```python
from build123d import *

# Parameters (mm, degrees)
SKETCH1_W                           = 250
SKETCH1_H                           = 250
SKETCH1_W_2                         = 4.8
SKETCH1_H_2                         = 20
SKETCH1_W_3                         = 10
SKETCH1_H_3                         = 2.9
SKETCH1_W_4                         = 2.9
SKETCH1_H_4                         = 30
SKETCH1_H_5                         = 50
SKETCH1_W_5                         = 6
SKETCH1_H_6                         = 70
BOSS_EXTRUDE1_DEPTH                 = 2
SKETCH2_R                           = 2.5
CUT_EXTRUDE1_DEPTH                  = 3
SKETCH3_R                           = 3.25
CUT_EXTRUDE2_DEPTH                  = 3
SKETCH4_W                           = 2
SKETCH4_H                           = 20
SKETCH4_W_2                         = 20
SKETCH4_H_2                         = 2
BOSS_EXTRUDE2_DEPTH                 = 2
F_4_5_4_5_DIAMETER_HOLE1_AT_2_COUNT = 2
F_4_5_4_5_DIAMETER_HOLE1_AT_2_PITCH = 50
F_4_5_4_5_DIAMETER_HOLE1_AT_3_COUNT = 2
F_4_5_4_5_DIAMETER_HOLE1_AT_3_PITCH = 130
F_4_5_4_5_DIAMETER_HOLE1_AT_4_COUNT = 2
F_4_5_4_5_DIAMETER_HOLE1_AT_4_PITCH = 120
SKETCH9_W                           = 4.8
SKETCH9_H                           = 20
CUT_EXTRUDE3_DEPTH                  = 3
SKETCH10_R                          = 2.1
CUT_EXTRUDE4_DEPTH                  = 5
SKETCH_1_R                          = 2.25
CUT_EXTRUDE_1_DEPTH                 = 2
CUT_EXTRUDE_1_DEPTH_BACK            = 10


with BuildPart() as part:
    # Sketch1 → Boss-Extrude1 (new body)
    with BuildSketch(Plane(origin=(0, 0, 0), x_dir=(1, 0, 0), z_dir=(0, 1, 0))):
        with Locations((125, 125)):
            Rectangle(SKETCH1_W, SKETCH1_H)
        with Locations((142.5, 15)):
            Rectangle(SKETCH1_W_2, SKETCH1_H_2, mode=Mode.SUBTRACT)
        with Locations((107.5, 15)):
            Rectangle(SKETCH1_W_2, SKETCH1_H_2, mode=Mode.SUBTRACT)
        with Locations((92, 53.93422616)):
            Rectangle(SKETCH1_W_3, SKETCH1_H_3, mode=Mode.SUBTRACT)
        with Locations((103.55, 79.434226159)):
            Rectangle(SKETCH1_W_4, SKETCH1_H_4, mode=Mode.SUBTRACT)
        with Locations((92, 104.93422616)):
            Rectangle(SKETCH1_W_3, SKETCH1_H_3, mode=Mode.SUBTRACT)
        with Locations((107.5, 125)):
            Rectangle(SKETCH1_W_2, SKETCH1_H_2, mode=Mode.SUBTRACT)
        with Locations((142.5, 125)):
            Rectangle(SKETCH1_W_2, SKETCH1_H_2, mode=Mode.SUBTRACT)
        with Locations((225, 200)):
            Rectangle(SKETCH1_W_2, SKETCH1_H_5, mode=Mode.SUBTRACT)
        with Locations((125, 135)):
            Rectangle(SKETCH1_W_5, SKETCH1_H_6, mode=Mode.SUBTRACT)
        with Locations((25, 200)):
            Rectangle(SKETCH1_W_2, SKETCH1_H_5, mode=Mode.SUBTRACT)
    extrude(amount=BOSS_EXTRUDE1_DEPTH)

    # Sketch2 → Cut-Extrude1 (cut, through all)
    with BuildSketch(Plane(origin=(0, 2, 0), x_dir=(1, 0, 0), z_dir=(0, 1, 0))):
        with Locations((15, 100)):
            Circle(SKETCH2_R)
        with Locations((63, 100)):
            Circle(SKETCH2_R)
    cut_extrude1 = extrude(amount=-CUT_EXTRUDE1_DEPTH, mode=Mode.SUBTRACT)

    # Sketch3 → Cut-Extrude2 (cut, through all)
    with BuildSketch(Plane(origin=(0, 2, 0), x_dir=(1, 0, 0), z_dir=(0, 1, 0))):
        with Locations((8, 8)):
            Circle(SKETCH3_R)
        with Locations((8, 237)):
            Circle(SKETCH3_R)
    cut_extrude2 = extrude(amount=-CUT_EXTRUDE2_DEPTH, mode=Mode.SUBTRACT)

    # Mirror1: Cut-Extrude2 across plane
    add(cut_extrude2.mirror(Plane.ZY.offset(-125)), mode=Mode.SUBTRACT)

    # Sketch4 → Boss-Extrude2 (add)
    with BuildSketch(Plane(origin=(0, 2, 0), x_dir=(1, 0, 0), z_dir=(0, 1, 0))):
        with Locations((-1, 190)):
            Rectangle(SKETCH4_W, SKETCH4_H)
        with Locations((-1, 60)):
            Rectangle(SKETCH4_W, SKETCH4_H)
        with Locations((60, -1)):
            Rectangle(SKETCH4_W_2, SKETCH4_H_2)
    boss_extrude2 = extrude(amount=-BOSS_EXTRUDE2_DEPTH)

    # Mirror2: Boss-Extrude2 across plane
    add(boss_extrude2.mirror(Plane.ZY.offset(-125)))

    # Mirror3: Cut-Extrude1 across plane
    add(cut_extrude1.mirror(Plane.ZY.offset(-125)), mode=Mode.SUBTRACT)

    # Sketch6 → Ø4.5 (4.5) Diameter Hole1 (revolve, cut)
    with BuildSketch(Plane(origin=(12.5, 2, -135), x_dir=(0, 0, 1), z_dir=(1, 0, 0))):
        Polygon((0, 0), (0, 11.351936393), (2.25, 10), (2.25, 0), align=None)
    f_4_5_4_5_diameter_hole1 = revolve(axis=Axis((12.5, 8.35, -135), (0, -1, 0)), mode=Mode.SUBTRACT)

    # Ø4.5 (4.5) Diameter Hole1 at 2: Ø4.5 (4.5) Diameter Hole1 ×2
    with Locations(*[(i * F_4_5_4_5_DIAMETER_HOLE1_AT_2_PITCH, 0, 0) for i in range(1, F_4_5_4_5_DIAMETER_HOLE1_AT_2_COUNT)]):
        add(f_4_5_4_5_diameter_hole1, mode=Mode.SUBTRACT)

    # Ø4.5 (4.5) Diameter Hole1 at 3: Ø4.5 (4.5) Diameter Hole1 ×2
    with Locations(*[Vector(0.384615385, 0, 0.923076923) * (i * F_4_5_4_5_DIAMETER_HOLE1_AT_3_PITCH) for i in range(1, F_4_5_4_5_DIAMETER_HOLE1_AT_3_COUNT)]):
        add(f_4_5_4_5_diameter_hole1, mode=Mode.SUBTRACT)

    # Ø4.5 (4.5) Diameter Hole1 at 4: Ø4.5 (4.5) Diameter Hole1 ×2
    with Locations(*[(0, 0, i * F_4_5_4_5_DIAMETER_HOLE1_AT_4_PITCH) for i in range(1, F_4_5_4_5_DIAMETER_HOLE1_AT_4_COUNT)]):
        add(f_4_5_4_5_diameter_hole1, mode=Mode.SUBTRACT)

    # Mirror4: Ø4.5 (4.5) Diameter Hole1 across plane
    add(f_4_5_4_5_diameter_hole1.mirror(Plane.ZY.offset(-125)), mode=Mode.SUBTRACT)

    # Mirror4 copy 1 sketch → Mirror4 copy 1 (revolve, cut)
    with BuildSketch(Plane(origin=(187.5, 2, -135), x_dir=(0, 0, 1), z_dir=(-1, 0, 0))):
        Polygon((0, 0), (0, -11.351936393), (2.25, -10), (2.25, 0), align=None)
    revolve(axis=Axis((187.5, 8.35, -135), (0, 1, 0)), mode=Mode.SUBTRACT)

    # Mirror4 copy 2 sketch → Mirror4 copy 2 (revolve, cut)
    with BuildSketch(Plane(origin=(187.5, 2, -15), x_dir=(0, 0, 1), z_dir=(-1, 0, 0))):
        Polygon((0, 0), (0, -11.351936393), (2.25, -10), (2.25, 0), align=None)
    revolve(axis=Axis((187.5, 8.35, -15), (0, 1, 0)), mode=Mode.SUBTRACT)

    # Mirror4 copy 3 sketch → Mirror4 copy 3 (revolve, cut)
    with BuildSketch(Plane(origin=(237.5, 2, -15), x_dir=(0, 0, 1), z_dir=(-1, 0, 0))):
        Polygon((0, 0), (0, -11.351936393), (2.25, -10), (2.25, 0), align=None)
    revolve(axis=Axis((237.5, 8.35, -15), (0, 1, 0)), mode=Mode.SUBTRACT)

    # Sketch9 → Cut-Extrude3 (cut, through all)
    with BuildSketch(Plane.XZ):
        with Locations((107.5, -185)):
            Rectangle(SKETCH9_W, SKETCH9_H)
    cut_extrude3 = extrude(amount=-CUT_EXTRUDE3_DEPTH, mode=Mode.SUBTRACT)

    # Mirror5: Cut-Extrude3 across plane
    add(cut_extrude3.mirror(Plane.ZY.offset(-125)), mode=Mode.SUBTRACT)

    # Sketch10 → Cut-Extrude4 (cut)
    with BuildSketch(Plane.XZ):
        with Locations((15, -210)):
            Circle(SKETCH10_R)
        with Locations((235, -210)):
            Circle(SKETCH10_R)
    extrude(amount=-CUT_EXTRUDE4_DEPTH, mode=Mode.SUBTRACT)

    # 草图1 → 切除-拉伸1 (cut, two sides)
    with BuildSketch(Plane(origin=(0, 0, 0), x_dir=(1, 0, 0), z_dir=(0, 1, 0))) as cut_extrude_1_sk:
        with Locations((38.4, 200)):
            Circle(SKETCH_1_R)
        with Locations((211.6, 200)):
            Circle(SKETCH_1_R)
    extrude(amount=CUT_EXTRUDE_1_DEPTH, mode=Mode.SUBTRACT)
    extrude(cut_extrude_1_sk.sketch, amount=-CUT_EXTRUDE_1_DEPTH_BACK, mode=Mode.SUBTRACT)


solid = part.part
```
The listing builds one solid part. Answer for the finished solid, in the listing's coordinates (mm). Coordinates: 2 decimals unless noted, no trailing zeros. Write each loop counter-clockwise with the first axis right and the second up, starting at its lowest first coordinate (ties: lowest second). Pieces come first, ordered by that corner, then holes. Notation, with made-up numbers: (-18, 23) -> (29, 23) arc R19 cw to (29, 27) -> close; hole circle Ø5 at (4.5, -32). An arc over 180 degrees is marked (long way). Write each question's results on one line, items separated by ' | '. Start each with the question number.
1) Flat-ended cylindrical pins translate along their axes: pin 1 Ø1 at (y, z) = (1, -205.5) entering from -X; pin 2 Ø1 at (y, z) = (1, -83.5) entering from +X; pin 3 Ø0.6 at (x, y) = (91.5, 1) entering from +Z. Find the tip coordinate at first contact, or state that the pin passes through.
2) A cutting plane is placed at B-B (z = -218). Determine the outline of the cut face in (x, y).
3) A cutting plane is placed at D-D (z = -190). Determine the outline of the cut face in (x, y).
4) A cutting plane is placed at A-A (z = -119). Determine the outline of the cut face in (x, y), then the cut area to 3 significant figures.
5) A cutting plane is placed at C-C (x = 125). Determine the outline of the cut face in (y, z).
6) Straight lines are drawn through the part: probe 1 along X at (y, z) = (0.6, -128.5); probe 2 along X at (y, z) = (1.45, -8); probe 3 along Z at (x, y) = (90, 0.8). For each, find the intervals that lie inside material, in ascending order.
7) For a pull along X with two mould halves and no side action, classify faces 1 (the cylindrical face through (244.395, 1.014, -239.197)), 2 (the flat face through (95, 0, -126)) as +X half, -X half, draft (parallel to the pull), parting line (faces both ways), or undercut.
Values follow:
1) pin 1: x = 0 | pin 2: x = 250 | pin 3: z = 0
2) outline: (0, 0) -> (22.6, 0) -> (22.6, 2) -> (0, 2) -> close; (27.4, 0) -> (222.6, 0) -> (222.6, 2) -> (27.4, 2) -> close; (227.4, 0) -> (250, 0) -> (250, 2) -> (227.4, 2) -> close
3) outline: (-2, 0) -> (22.6, 0) -> (22.6, 2) -> (-2, 2) -> close; (27.4, 0) -> (105.1, 0) -> (105.1, 2) -> (27.4, 2) -> close; (109.9, 0) -> (140.1, 0) -> (140.1, 2) -> (109.9, 2) -> close; (144.9, 0) -> (222.6, 0) -> (222.6, 2) -> (144.9, 2) -> close; (227.4, 0) -> (252, 0) -> (252, 2) -> (227.4, 2) -> close
4) outline: (0, 0) -> (105.1, 0) -> (105.1, 2) -> (0, 2) -> close; (109.9, 0) -> (122, 0) -> (122, 2) -> (109.9, 2) -> close; (128, 0) -> (140.1, 0) -> (140.1, 2) -> (128, 2) -> close; (144.9, 0) -> (250, 0) -> (250, 2) -> (144.9, 2) -> close | area: 469 mm²
5) outline: (0, -250) -> (2, -250) -> (2, -170) -> (0, -170) -> close; (0, -100) -> (2, -100) -> (2, 0) -> (0, 0) -> close
6) probe 1: 0 to 105.1, 109.9 to 122, 128 to 140.1, 144.9 to 250 | probe 2: 0 to 4.75, 11.25 to 105.1, 109.9 to 140.1, 144.9 to 238.75, 245.25 to 250 | probe 3: -250 to -106.38, -103.48 to -55.38, -52.48 to 0
7) face 1: undercut | face 2: draft
